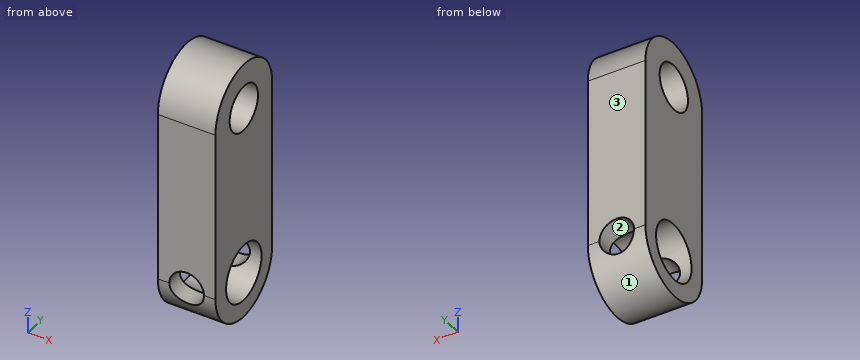
from build123d import *

# Parameters (mm, degrees)
SKETCH_1_R          = 4
SKETCH_1_R_2        = 5
EXTRUDE_1_DEPTH     = 10
SKETCH_2_R          = 3
CUT_EXTRUDE_1_DEPTH = 17


with BuildPart() as part:
    # 草图1 → 凸台-拉伸1 (new body)
    with BuildSketch(Plane(origin=(0, 0, 0), x_dir=(0, 0, -1), z_dir=(1, 0, 0))):
        with BuildLine():
            Line((15, 8), (-15, 8))
            ThreePointArc((-15, 8), (-23, 0), (-15, -8))
            Line((-15, -8), (15, -8))
            ThreePointArc((15, -8), (23, 0), (15, 8))
        make_face()
        with Locations((-15, 0)):
            Circle(SKETCH_1_R, mode=Mode.SUBTRACT)
        with Locations((15, 0)):
            Circle(SKETCH_1_R_2, mode=Mode.SUBTRACT)
    extrude(amount=EXTRUDE_1_DEPTH)

    # 草图2 → 切除-拉伸1 (cut, through all)
    with BuildSketch(Plane(origin=(0, 8, 0), x_dir=(1, 0, 0), z_dir=(0, 1, 0))):
        with Locations((5, 15)):
            Circle(SKETCH_2_R)
    extrude(amount=-CUT_EXTRUDE_1_DEPTH, mode=Mode.SUBTRACT)


solid = part.part
Geometry check sheet. Reference: the model listing, model coordinates, mm. Face numbers are marked on the shaded views. Round coordinates to 2 decimals unless told otherwise and drop trailing zeros. Loops run counter-clockwise (first coordinate to the right, second up) from the corner with the lowest first, then second, coordinate; pieces in that order, holes last. Notation, with made-up numbers: (-30.5, 58.25) -> (6.5, 58.25) arc R17 ccw to (6.5, 80.25) -> close; hole circle Ø10 at (-20.5, -4.5). An arc over 180 degrees is marked (long way). Answer as a JSON object with one key per item and string values. Group by question number.
Item 1: Cross-section at C-C, the plane z = 13. Record the cut outline in (x, y), plus the area to 3 significant figures.
Item 2: Cross-section at D-D, the plane x = 9. Record the cut outline in (y, z).
Item 3: Cross-section at B-B, the plane x = 5. Record the cut outline in (y, z), plus the area to 3 significant figures.
Item 4: Thickness scan on line 1 along Y through (x, z) = (6.75, -12); line 2 along X through (y, z) = (6.1, -15); line 3 along Z through (x, y) = (6, 2.25). Record the ranges inside material, lowest first.
Item 5: Release check for a two-part mould opening along Z. For the marked faces 1, 2 and 3 record: pulls with the +Z half, pulls with the -Z half, needs draft (parallel to the pull), parting line crosses it, or undercut.
Item 6: Cross-section at A-A, the plane y = 0. Record the cut outline in (x, z).
Item 7: Depth check by flat-ended pin: pin 1 Ø4 at (x, y) = (3.5, -4) entering from -Z; pin 2 Ø1 at (x, z) = (3, 17.5) entering from -Y. Enter the tip coordinate at first touch or a pass-through.
Determined:
{
 "1": {"outline": "(0, -8) -> (10, -8) -> (10, -3.46) -> (0, -3.46) -> close; (0, 3.46) -> (10, 3.46) -> (10, 8) -> (0, 8) -> close", "area": "90.7 mm²"},
 "2": {"outline": "(-8, -15) arc R8 ccw to (8, -15) -> (8, 15) arc R8 ccw to (-8, 15) -> close; hole circle Ø10 at (0, -15); hole circle Ø8 at (0, 15)"},
 "3": {"outline": "(-8, -12) -> (-4, -12) arc R5 cw to (4, -12) -> (8, -12) -> (8, 15) arc R8 ccw to (-8, 15) -> close; (-7.42, -18) arc R8 ccw to (7.42, -18) -> (4, -18) arc R5 cw to (-4, -18) -> close; hole circle Ø8 at (0, 15)", "area": "514 mm²"},
 "4": {"line 1": "y = -8 to -4, 4 to 8", "line 2": "x = 0 to 2, 8 to 10", "line 3": "z = -22.68 to -19.47, -10.53 to 11.69, 18.31 to 22.68"},
 "5": {"face 1": "pulls with the -Z half", "face 2": "undercut", "face 3": "needs draft"},
 "6": {"outline": "(0, -23) -> (10, -23) -> (10, -20) -> (0, -20) -> close; (0, -10) -> (10, -10) -> (10, 11) -> (0, 11) -> close; (0, 19) -> (10, 19) -> (10, 23) -> (0, 23) -> close"},
 "7": {"pin 1": "stops at z = -22.75", "pin 2": "stops at y = -7.75"}
}
